The listing builds one solid part. Answer for the finished solid, in the listing's coordinates (mm). A direction names the side the tool comes from. Round coordinates to 2 decimals unless told otherwise and drop trailing zeros. Write each loop counter-clockwise with the first axis right and the second up, starting at its lowest first coordinate (ties: lowest second). Pieces come first, ordered by that corner, then holes. Notation, with made-up numbers: (-37, 22) - (-27, 22) arc R14 cw to (-27, 48) - close; hole circle Ø6 at (47, 67). An arc over 180 degrees is marked (long way). Return JSON: item names as keys, results as strings. Group by question number.
from build123d import *

# Parameters (mm, degrees)
EXTRUDE_1_DEPTH     = 5
SKETCH_2_R          = 3.75
CUT_EXTRUDE_1_DEPTH = 6
FILLET_1_R          = 10
SKETCH_3_W          = 22
SKETCH_3_H          = 25
CUT_EXTRUDE_2_DEPTH = 6
FILLET_2_R          = 2


with BuildPart() as part:
    # ｽｹｯﾁ1 → ﾎﾞｽ - 押し出し1 (new body)
    with BuildSketch(Plane(origin=(0, 0, 0), x_dir=(1, 0, 0), z_dir=(0, 1, 0))):
        Polygon((-50, 38.5), (-50, 50), (-38.5, 50), (-23.5, 35), (23.5, 35), (38.5, 50), (50, 50), (50, 38.5), (35, 23.5), (35, -23.5), (50, -38.5), (50, -50), (38.5, -50), (23.5, -35), (-23.5, -35), (-38.5, -50), (-50, -50), (-50, -38.5), (-35, -23.5), (-35, 23.5), align=None)
    extrude(amount=EXTRUDE_1_DEPTH)

    # ｽｹｯﾁ2 → ｶｯﾄ - 押し出し1 (cut, through all)
    with BuildSketch(Plane(origin=(0, 5, 0), x_dir=(1, 0, 0), z_dir=(0, 1, 0))):
        with Locations((-39, 39)):
            Circle(SKETCH_2_R)
        with Locations((39, 39)):
            Circle(SKETCH_2_R)
        with Locations((39, -39)):
            Circle(SKETCH_2_R)
        with Locations((-39, -39)):
            Circle(SKETCH_2_R)
    extrude(amount=-CUT_EXTRUDE_1_DEPTH, mode=Mode.SUBTRACT)

    # ﾌｨﾚｯﾄ1
    fillet_1_edges = [part.edges().sort_by_distance(p)[0] for p in [
        (-23.5, 2.5, -35),
        (23.5, 2.5, -35),
        (35, 2.5, -23.5),
        (35, 2.5, 23.5),
        (23.5, 2.5, 35),
        (-23.5, 2.5, 35),
        (-35, 2.5, 23.5),
        (-35, 2.5, -23.5),
    ]]
    fillet(fillet_1_edges, radius=FILLET_1_R)

    # ｽｹｯﾁ3 → ｶｯﾄ - 押し出し2 (cut, through all)
    with BuildSketch(Plane(origin=(0, 5, 0), x_dir=(1, 0, 0), z_dir=(0, 1, 0))):
        Rectangle(SKETCH_3_W, SKETCH_3_H)
    extrude(amount=-CUT_EXTRUDE_2_DEPTH, mode=Mode.SUBTRACT)

    # ﾌｨﾚｯﾄ2
    fillet_2_edges = [part.edges().sort_by_distance(p)[0] for p in [
        (11, 2.5, -12.5),
        (11, 2.5, 12.5),
        (-11, 2.5, 12.5),
        (-11, 2.5, -12.5),
    ]]
    fillet(fillet_2_edges, radius=FILLET_2_R)


solid = part.part
(1) For faces 5 (the cylindrical face through (35.74, 2.54, 23.13)), 6 (the cylindrical face through (23.13, 2.54, -35.74)), 7 (the flat face through (-44, 2.5, 32.5)), 8 (the flat face through (0, 3, 12.5)), determine the directions among +Z, -Z, +X, -X, +Y, -Y from which every point of the face is accessible in a straight line to the end or side of a thin tool.
(2) Consider line 1 (X direction, y = 1.3, z = 39); line 2 (X direction, y = 3.7, z = -39.5); line 3 (Z direction, x = 5.5, y = 0.65). Determine where each line is inside the solid, lowest interval first.
(3) Determine the mould class of faces 1 (the flat face through (-44, 2, -50)), 2 (the cylindrical face through (-23.235, 2.535, 35.782)), 3 (the cylindrical face through (36.024, 2.535, 41.282)), 4 (the flat face through (-35, 2, 0)) for opening direction X: +X half, -X half, draft (parallel to the pull), parting line (faces both ways), or undercut.
(4) Find section C-C (z = 31.5). Write down the section's boundary in (x, y), plus the area to 3 significant figures.
(5) Find section D-D (y = 3.85). State how many separate pieces and enclosed holes the cut face has, plus the area to 3 significant figures.
(6) Find section B-B (x = -31.5). Write down the section's boundary in (y, z).
(7) Find section A-A (z = 6). Write down the section's boundary in (x, y).
(8) Flat-ended cylindrical pins translate along their axes: pin 1 (1 mm diameter, centred on x = -16, y = 3, fed in from -Z); pin 2 (10 mm diameter, centred on x = -39, z = 39, fed in from -Y); pin 3 (1.5 mm diameter, centred on x = -1, y = 2, fed in from +Z); pin 4 (2 mm diameter, centred on y = 2, z = 20.5, fed in from +X). Find the tip coordinate at first contact, or state that the pin passes through.
Check sheet entries:
{
 "1": {"face 5": "+X, +Y, -Y", "face 6": "-Z, +Y, -Y", "face 7": "-X, +Y, -Y", "face 8": "+Y, -Y"},
 "2": {"line 1": "x = -50 to -42.75, -35.25 to -27.5, 27.5 to 35.25, 42.75 to 50", "line 2": "x = -50 to -42.72, -35.28 to -28, 28 to 35.28, 42.72 to 50", "line 3": "z = -35 to -12.5, 12.5 to 35"},
 "3": {"face 1": "draft", "face 2": "undercut", "face 3": "undercut", "face 4": "-X half"},
 "4": {"outline": "(-43, 0) - (43, 0) - (43, 5) - (-43, 5) - close", "area": "430 mm^2"},
 "5": {"separate pieces": "1", "enclosed holes": "5", "area": "5,570 mm^2"},
 "6": {"outline": "(0, -43) - (5, -43) - (5, 43) - (0, 43) - close"},
 "7": {"outline": "(-35, 0) - (-11, 0) - (-11, 5) - (-35, 5) - close; (11, 0) - (35, 0) - (35, 5) - (11, 5) - close"},
 "8": {"pin 1": "stops at z = -35", "pin 2": "stops at y = 0", "pin 3": "stops at z = 35", "pin 4": "stops at x = 35.23"}
}
